from build123d import *

# Parameters (mm, degrees)
F0_W          = 5.842
F0_H          = 12.7
F0_R          = 3.175
F2_DEPTH      = 3.175
F3_R          = 1.524
F4_DEPTH      = 6.35
F4_DEPTH_BACK = 1.27
F6_R          = 1.524
F7_DEPTH      = 17.78
F5_R          = 1.524
F8_DEPTH      = 10.414
F9_DEPTH      = 56.134
F10_R         = 1.27


with BuildPart() as f1:
    # F0 (on Front) → F1 (revolve)
    with BuildSketch(Plane.XZ):
        Polygon((5.842, 12.7), (5.842, 0), (66.294, 0), (66.294, 12.7), (56.134, 12.7), (56.134, 10.16), (10.16, 10.16), (10.16, 12.7), align=None)
        with Locations((2.921, 6.35)):
            Rectangle(F0_W, F0_H)
    revolve(axis=Axis((33.147, 0, 0), (-1, 0, 0)))

    # F0 (on Front) → F2 (join, symmetric)
    with BuildSketch(Plane.XZ):
        with Locations((2.921, 6.35)):
            Rectangle(F0_W, F0_H)
        with BuildLine():
            Line((-0.9398, 0), (0, 0))
            Line((0, 0), (0, 12.7))
            Line((0, 12.7), (5.842, 12.7))
            Line((5.842, 12.7), (5.842, 15.24))
            Line((5.842, 15.24), (-0.508, 15.24))
            Line((-0.508, 15.24), (-10.88063, 3.847543))
            ThreePointArc((-10.88063, 3.847543), (-4.591961, 5.329721), (-0.9398, 0))
        make_face()
        with BuildLine():
            ThreePointArc((-8.182663, -5.506983), (-3.195791, -4.549339), (-0.9398, 0))
            ThreePointArc((-0.9398, 0), (-4.591961, 5.329721), (-10.88063, 3.847543))
            ThreePointArc((-10.88063, 3.847543), (-12.145978, -1.583727), (-8.182663, -5.506983))
        make_face()
        with Locations((-6.6548, 0)):
            Circle(F0_R, mode=Mode.SUBTRACT)
        with BuildLine():
            Line((5.842, 0), (0, 0))
            Line((0, 0), (-0.9398, 0))
            ThreePointArc((-0.9398, 0), (-3.195791, -4.549339), (-8.182663, -5.506983))
            Line((-8.182663, -5.506983), (5.842, -9.398))
            Line((5.842, -9.398), (5.842, 0))
        make_face()
    extrude(amount=F2_DEPTH, both=True)

    # F3 (on face) → F4 (join, two sides)
    with BuildSketch(Plane.YZ.offset(66.294)) as f4_sk:
        with BuildLine():
            ThreePointArc((-5.08, 0), (0, -5.08), (5.08, 0))
            ThreePointArc((5.08, 0), (0, 5.08), (-5.08, 0))
        make_face()
        Circle(F3_R, mode=Mode.SUBTRACT)
        with BuildLine():
            ThreePointArc((-5.08, 0), (0, 5.08), (5.08, 0))
            Line((5.08, 0), (5.08, 15.24))
            Line((5.08, 15.24), (-5.08, 15.24))
            Line((-5.08, 15.24), (-5.08, 0))
        make_face()
    extrude(amount=F4_DEPTH)
    extrude(f4_sk.sketch, amount=-F4_DEPTH_BACK)

    # F6 (on face) → F7 (cut)
    with BuildSketch(Plane.XY.offset(15.24)):
        with Locations((2.667, 0)):
            Circle(F6_R)
    extrude(amount=-F7_DEPTH, mode=Mode.SUBTRACT)

    # F5 (on face) → F8 (cut)
    with BuildSketch(Plane.XY.offset(15.24)):
        with Locations((68.834, 0)):
            Circle(F5_R)
    extrude(amount=-F8_DEPTH, mode=Mode.SUBTRACT)

    # F3 (on face) → F9 (cut, through all)
    with BuildSketch(Plane.YZ.offset(66.294)):
        Circle(F3_R)
    extrude(amount=-F9_DEPTH, mode=Mode.SUBTRACT)

    # F10
    f10_edges = [f1.edges().sort_by_distance(p)[0] for p in [
        (65.024, 5.08, 13.439871),
        (65.024, 0, 15.24),
        (68.834, 5.08, 15.24),
        (72.644, 0, 15.24),
        (68.834, -5.08, 15.24),
        (72.644, 5.08, 7.62),
        (72.644, -5.08, 7.62),
        (2.667, 3.175, 15.24),
        (-5.694315, 3.175, 9.543772),
        (5.842, 0, 15.24),
        (2.667, -3.175, 15.24),
        (5.842, -3.175, 13.768361),
        (-0.508, 0, 15.24),
        (-5.694315, -3.175, 9.543772),
    ]]
    fillet(f10_edges, radius=F10_R)


solid = f1.part
Can you work these out from the model? Positions are in its coordinate system, mm. A direction names the side the tool comes from. Round coordinates to 2 decimals unless told otherwise and drop trailing zeros. Loops run counter-clockwise (first coordinate to the right, second up) from the corner with the lowest first, then second, coordinate; pieces in that order, holes last. Notation, with made-up numbers: (-18.5, 37) - (26.5, 37) arc R6 ccw to (26.5, 43) - close; hole circle Ø8 at (-33.5, 2). An arc over 180 degrees is marked (long way). Answer in a Markdown table with one row per item. Add a question column.
Q1. I want a section at A-A on x = 9. List the corners of the cut face in (y, z) for me.
Q2. I want a section at B-B on x = 25. List the corners of the cut face in (y, z) for me, and give its area (3 significant figures).
Q3. I want a section at C-C on y = 8.75. List the corners of the cut face in (x, z) for me, and give its area (3 significant figures).
Q4. I need wall thicknesses on L1, parallel to X at y = 5.25, z = 11.25; L2, parallel to X at y = -6.5, z = -7.5; L3, parallel to X at y = 0.5, z = 2.5. Which ranges of each line are inside material? Lowest first, please.
Q5. We'd pull the mould along Z, two halves only. Please class faces 5 (the cylindrical face through (68.8, -0.11, -5.08)), 6 (the cylindrical face through (-3.626, 0.044, 0.954)), 7 (the flat face through (10.16, 9, 6)), 8 (the cylindrical face through (5.01, -12.4, -2.75)): pulls with the +Z half, pulls with the -Z half, needs draft (parallel to the pull), parting line crosses it, or undercut.
Q6. Which directions (+Z, -Z, +X, -X, +Y, -Y) give clear straight access to the entire face, cutting with the end or side of a thin tool? Please do faces 1 (the cylindrical face through (70.288, 0.458, 10.106)), 2 (the flat face through (0, -5, 0)), 3 (the flat face through (69, 5.08, 7)), 4 (the flat face through (66.294, 0, -6)).
Q7. For pin 1 Ø8.5 at (x, z) = (1, 7.5) entering from +Y; pin 2 Ø8 at (x, y) = (55.5, -2.5) entering from +Z; pin 3 Ø1.5 at (x, y) = (28, -3) entering from -Z; pin 4 Ø8 at (x, z) = (0, 1) entering from -Y, each with a flat end and sliding along its axis, tell me the tip position at first contact or that it passes through.
A:
| question | item | result |
|---|---|---|
| 1 | outline | circle Ø25.4 at (0, 0) |
| 2 | outline | circle Ø20.32 at (0, 0); hole circle Ø3.05 at (0, 0) |
| 2 | area | 317 mm^2 |
| 3 | outline | (0, -9.2) - (10.16, -9.2) - (10.16, -5.16) - (56.13, -5.16) - (56.13, -9.2) - (66.29, -9.2) - (66.29, 9.2) - (56.13, 9.2) - (56.13, 5.16) - (10.16, 5.16) - (10.16, 9.2) - (0, 9.2) - close |
| 3 | area | 849 mm^2 |
| 4 | L1 | 0 to 10.16, 56.13 to 66.29 |
| 4 | L2 | 0 to 66.29 |
| 4 | L3 | -11.79 to -8.61, -4.7 to 1.23, 4.11 to 72.64 |
| 5 | face 5 | pulls with the -Z half |
| 5 | face 6 | undercut |
| 5 | face 7 | needs draft |
| 5 | face 8 | parting line crosses it |
| 6 | face 1 | +Z |
| 6 | face 2 | -Z, -X |
| 6 | face 3 | +Z, -Z, +X, +Y |
| 6 | face 4 | -Z, +X |
| 7 | pin 1 | y = 12.28 |
| 7 | pin 2 | z = 12.7 |
| 7 | pin 3 | z = -9.91 |
| 7 | pin 4 | y = -12.7 |
